Work out the finished part from the listing and answer in its coordinate system (mm). A direction names the side the tool comes from. Coordinates: 2 decimals unless noted, no trailing zeros. Write each loop counter-clockwise with the first axis right and the second up, starting at its lowest first coordinate (ties: lowest second). Pieces come first, ordered by that corner, then holes. Notation, with made-up numbers: M 65.5,30.25 L 102.5,30.25 A21 ccw 102.5,49.25 Z; hole C -40,21.25 d6. An arc over 180 degrees is marked long. Use CSV: the item, a comma, the result in double quotes.
Autodesk Inventor part; units mm, degrees
ref_plane "Work Plane1" through (-6.35, 0, 0) normal (1, 0, 0) x (0, 1, 0)
ref_plane "YZ Plane" through (0, 0, 0) normal (1, 0, 0) x (0, 1, 0)
ref_plane "XZ Plane" through (0, 0, 0) normal (0, 1, 0) x (-1, 0, 0)
sketch "Sketch1" plane through (0, 0, 0) normal (0, 0, 1) x (1, 0, 0)
  circle A0 centre (0, 0) radius 6.35
  dimension "d0" = 12.7
extrude "Extrusion1" add sketch "Sketch1" along normal mid plane 76.2
sketch "Sketch2" plane through (0, 0, 38.1) normal (0, 0, 1) x (1, 0, 0)
  circle A0 centre (0, 0) radius 6.35
  circle A1 centre (0, 0) radius 5
  dimension "d3" = 10
extrude "Extrusion2" add sketch "Sketch2" along normal blind 19 contours A1
sketch "Sketch3" plane through (0, 0, 57.1) normal (0, 0, 1) x (1, 0, 0)
  circle A0 centre (0, 0) radius 5
  line L0 (-4, 3) -> (-4, -3)
  line L1 (4, 3) -> (4, -3)
  line L2 (4, 0) -> (5, 0) construction
  line L3 (-4, 0) -> (-5, 0) construction
  dimension "d7" = 8
extrude "Extrusion3" cut sketch "Sketch3" against normal blind 4 contours A0 L1 | L0 A0
sketch "Sketch4" plane through (0, 0, -38.1) normal (0, 0, -1) x (-1, 0, 0)
  circle A0 centre (0, 0) radius 6.35
hole "Hole1" at (0, 0, -38.1) direction (0, 0, 1) diameter 2.85 depth 19 tip angle 118
chamfer "Chamfer1" distance 0.25 angle 45 3 edges at (0, -1.425, -38.1) (-6.35, 0, -38.1) (-6.35, 0, 38.1)
ref_plane "Work Plane1" through (-6.35, 0, 0) normal (1, 0, 0) x (0, 1, 0)
sketch "Sketch5" plane through (-6.35, 0, 0) normal (1, 0, 0) x (0, 1, 0)
  line L0 (6.1, -38.1) -> (-6.1, -38.1)
  line L1 (0, -38.1) -> (0, 22.7756) construction
  arc A0 (1.5875, 26.9) -> (-1.5875, 26.9) centre (0, 26.9) ccw
  line L2 (1.5875, -38.1) -> (1.5875, 26.9)
  line L3 (-1.5875, 26.9) -> (-1.5875, -38.1)
  dimension "d20" = 3.175
  dimension "d25" = 65
extrude "Extrusion4" cut sketch "Sketch5" along normal blind 1.5875
properties part number "BB1-Axle" material "Steel, Mild"
Item 1: Given pin 1 (1.1 mm diameter, centred on x = -5.5, z = 1, fed in from +Y); pin 2 (2 mm diameter, centred on y = 2, z = -9, fed in from -X); pin 3 (5 mm diameter, centred on y = 5, z = 43, fed in from +X), each flat-ended and moving along its own axis, determine where each tip first touches the part or whether it passes through.
Answer:
pin 1,"stops at y = 3.98"
pin 2,"stops at x = -6.15"
pin 3,"stops at x = 4.33"
Item 2: The part is cut by section B-B (z = 49). Write down the section's boundary in (x, y), then the cut area to 3 significant figures.
Answer:
outline,"C 0,0 d10"
area,"78.5 mm2"
Item 3: For a pull along X with two mould halves and no side action, classify faces 1 (the face through (-5, 2, 38.1)), 2 (the face through (-5, 0, 47)), 3 (the face through (0.87, -1.13, -28.34)), 4 (the face through (-0.24, -0.05, -18.39)) as released by +X, released by -X, zero draft, split by the parting line, or undercut.
Answer:
face 1,"zero draft"
face 2,"split by the parting line"
face 3,"undercut"
face 4,"undercut"
Item 4: A tool of negligible diameter and unlimited length cuts with its end or side. For faces 5 (the face through (4, 0, 55)), 6 (the face through (-4, 0, 55)), 7 (the face through (0, 0, 57.1)), 8 (the face through (6.057, 1.907, 0.53)), 9 (the face through (-4.762, 0, -4)), from which of +Z, -Z, +X, -X, +Y, -Y can it reach the whole face along a straight path? Write none if from no direction.
Answer:
face 5,"+Z, +X, +Y, -Y"
face 6,"+Z, -X, +Y, -Y"
face 7,"+Z, +X, -X, +Y, -Y"
face 8,"+Z, -Z"
face 9,"-Z, -X"
Item 5: The part is cut by section C-C (z = -8). Write down the section's boundary in (x, y), then the cut area to 3 significant figures.
Answer:
outline,"M -6.15,-1.59 A6.35 ccw long -6.15,1.59 L -4.76,1.59 L -4.76,-1.59 Z"
area,"122 mm2"
Item 6: Consider probe 1 along Y at (x, z) = (0, -28.5) (3 decimals); probe 2 along Y at (x, z) = (-5.25, 20); probe 3 along Z at (x, y) = (-2.5, 5.5). Determine where each line is inside the solid, lowest interval first.
Answer:
probe 1,"y = -6.35 to -1.425, 1.425 to 6.35"
probe 2,"y = -3.57 to -1.59, 1.59 to 3.57"
probe 3,"z = -38.1 to 38.1"
